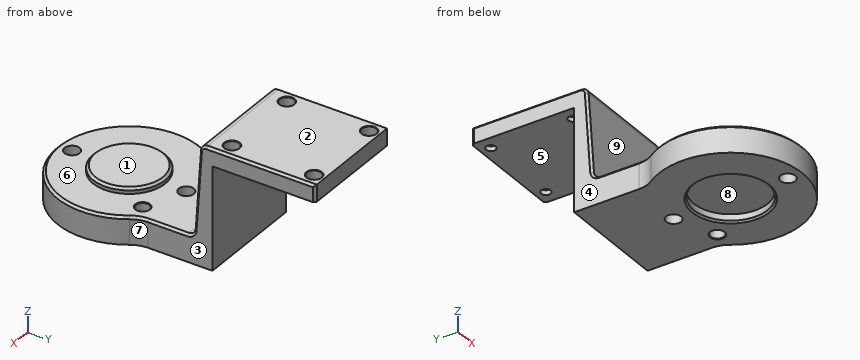
```python
from build123d import *

# Parameters (mm, degrees)
SKETCH_R          = 31.4
PAD_DEPTH         = 12
SKETCH001_R       = 16.15
PAD001_DEPTH      = 2.5
SKETCH009_R       = 15.75
PAD004_DEPTH      = 2.5
PAD001_FACE4_R    = 16.15
POCKET_DEPTH      = 3.5
SKETCH002_R       = 3.3
POCKET001_DEPTH   = 20
CHAMFER_SIZE      = 1
CHAMFER001_SIZE   = 0.75
SKETCH003_R       = 3
POCKET002_DEPTH   = 12
CHAMFER003_SIZE   = 0.25
PAD005_DEPTH      = 12
PAD006_DEPTH      = 24
PAD006_DEPTH_BACK = 24
SKETCH012_R       = 2.1
POCKET003_DEPTH   = 9.420822
SKETCH013_R       = 3.2
POCKET004_DEPTH   = 5.35
FILLET_R          = 12
FILLET001_R       = 3
CHAMFER004_SIZE   = 1
CHAMFER005_SIZE   = 1
CHAMFER006_SIZE   = 0.2


with BuildPart() as part:
    # Sketch → Pad (new body)
    with BuildSketch(Plane.XY):
        Circle(SKETCH_R)
    extrude(amount=PAD_DEPTH)

    # Sketch001 (on Sketch) → Pad001 (join)
    with BuildSketch(Plane.XY):
        Circle(SKETCH001_R)
    extrude(amount=PAD001_DEPTH)

    # Sketch009 (on Face3 of Pad001) → Pad004 (join)
    with BuildSketch(Plane.XY.offset(12)):
        Circle(SKETCH009_R)
    extrude(amount=PAD004_DEPTH)

    # Pad001 Face4 → Pocket (cut)
    with BuildSketch(Plane(origin=(0, 0, 0), x_dir=(0, -1, 0), z_dir=(0, 0, -1))):
        Circle(PAD001_FACE4_R)
    extrude(amount=-POCKET_DEPTH, mode=Mode.SUBTRACT)

    # Sketch002 → Pocket001 (cut)
    with BuildSketch(Plane.XY):
        with Locations((0, 25)):
            Circle(SKETCH002_R)
        with Locations((0, -25)):
            Circle(SKETCH002_R)
    extrude(amount=POCKET001_DEPTH, mode=Mode.SUBTRACT)

    # Chamfer
    chamfer_edges = [part.edges().sort_by_distance(p)[0] for p in [
        (-15.75, 0, 14.5),
    ]]
    chamfer(chamfer_edges, length=CHAMFER_SIZE)

    # Chamfer001
    chamfer001_edges = [part.edges().sort_by_distance(p)[0] for p in [
        (-16.15, 0, 0),
    ]]
    chamfer(chamfer001_edges, length=CHAMFER001_SIZE)

    # Sketch003 (on Face7 of Chamfer001) → Pocket002 (cut)
    with BuildSketch(Plane.XY.offset(12)):
        with Locations((17.67767, 17.67767)):
            Circle(SKETCH003_R)
    extrude(amount=-POCKET002_DEPTH, mode=Mode.SUBTRACT)

    # Chamfer003
    chamfer003_edges = [part.edges().sort_by_distance(p)[0] for p in [
        (14.67767, 17.67767, 12),
        (14.67767, 17.67767, 0),
    ]]
    chamfer(chamfer003_edges, length=CHAMFER003_SIZE)

    # Sketch011 → Pad005 (join)
    with BuildSketch(Plane.XY):
        with BuildLine():
            Line((24, 20.247469), (24, 34.174057))
            Line((24, 34.174057), (-24, 34.174057))
            Line((-24, 34.174057), (-24, 20.247469))
            ThreePointArc((24, 20.247469), (0, 31.4), (-24, 20.247469))
        make_face()
    extrude(amount=PAD005_DEPTH)

    # Sketch010 → Pad006 (join, two sides)
    with BuildSketch(Plane.YZ) as pad006_sk:
        Polygon((34.020989, 0), (52.498643, 0), (52.498643, 45), (97.498643, 45), (97.498643, 52.420822), (47.04097, 52.420822), (44.319458, 12), (34.020989, 12), align=None)
    extrude(amount=PAD006_DEPTH)
    extrude(pad006_sk.sketch, amount=-PAD006_DEPTH_BACK)

    # Sketch012 (on Face31 of Pad006) → Pocket003 (cut)
    with BuildSketch(Plane(origin=(0, 0, 45), x_dir=(1, 0, 0), z_dir=(0, 0, -1))):
        with Locations((18, -92.99873)):
            Circle(SKETCH012_R)
        with Locations((-18, -92.99873)):
            Circle(SKETCH012_R)
        with Locations((-18, -56.99873)):
            Circle(SKETCH012_R)
        with Locations((18, -56.99873)):
            Circle(SKETCH012_R)
    extrude(amount=-POCKET003_DEPTH, mode=Mode.SUBTRACT)

    # Sketch013 (on Face29 of Pocket003) → Pocket004 (cut)
    with BuildSketch(Plane.XY.offset(52.420822)):
        with Locations((18, 93.000084)):
            Circle(SKETCH013_R)
        with Locations((-18, 93.000084)):
            Circle(SKETCH013_R)
        with Locations((-18, 57.000084)):
            Circle(SKETCH013_R)
        with Locations((18, 57.000084)):
            Circle(SKETCH013_R)
    extrude(amount=-POCKET004_DEPTH, mode=Mode.SUBTRACT)

    # Fillet
    fillet_edges = [part.edges().sort_by_distance(p)[0] for p in [
        (-24, 20.247469, 6),
        (24, 20.247469, 6),
    ]]
    fillet(fillet_edges, radius=FILLET_R)

    # Fillet001
    fillet001_edges = [part.edges().sort_by_distance(p)[0] for p in [
        (0, 44.319458, 12),
        (0, 47.04097, 52.420822),
    ]]
    fillet(fillet001_edges, radius=FILLET001_R)

    # Chamfer004
    chamfer004_edges = [part.edges().sort_by_distance(p)[0] for p in [
        (24, 29.130313, 12),
        (-24, 29.130313, 12),
    ]]
    chamfer(chamfer004_edges, length=CHAMFER004_SIZE)

    # Chamfer005
    chamfer005_edges = [part.edges().sort_by_distance(p)[0] for p in [
        (24, 97.498643, 48.210411),
        (-24, 97.498643, 48.210411),
    ]]
    chamfer(chamfer005_edges, length=CHAMFER005_SIZE)

    # Chamfer006
    chamfer006_edges = [part.edges().sort_by_distance(p)[0] for p in [
        (-21.2, 57.000084, 52.420822),
        (-21.2, 93.000084, 52.420822),
        (14.8, 93.000084, 52.420822),
        (14.8, 57.000084, 52.420822),
    ]]
    chamfer(chamfer006_edges, length=CHAMFER006_SIZE)


solid = part.part
```
Input: part model. Units: mm. Frame: model coordinates. Face numbers are marked on the shaded views. A direction names the side the tool comes from. Give positions to 0.01 mm unless a question says otherwise; leave off trailing zeros. Order: outer loops, then holes, each group sorted by start corner. A loop starts at its lowest first (then second) coordinate and runs counter-clockwise, first axis right, second up. Notation, with made-up numbers: (22.5, -17) -> (26.5, -17) arc R13 cw to (26.5, 4) -> close; hole circle Ø1 at (16, 38.25). An arc over 180 degrees is marked (long way). Write each question's results on one line, items separated by ' | '. Start each with the question number.
Item 1: Cut plane A-A on y = 0. Return the cut outline in (x, z).
Item 2: Contact query for flat-ended pins moving along their axis: P1, Ø5, axis at x = 18, y = 57, coming from the -Z side; P2, Ø12, axis at x = 24.5, z = 19.5, coming from the -Y side; P3, Ø5, axis at x = 19.5, y = 56, coming from the +Z side; P4, Ø4, axis at x = -16.5, z = 17, coming from the -Y side. Output: stop coordinate, or through.
Item 3: Line query: line 1 (Y direction, x = -18, z = 50); line 2 (Z direction, x = 23, y = 12); line 3 (Y direction, x = -18, z = 45.8). Output: solid intervals per line, ascending.
Item 4: Cut plane D-D on y = 64.5. Return the cut outline in (x, z), then the cut area to 3 significant figures.
Item 5: Set-up query: the marked faces 1, 2, 3, 4 and 5. Return all of +Z, -Z, +X, -X, +Y, -Y with unobstructed straight access to the full face (end or side cutting, diameter ignored); none if empty.
Item 6: Cut plane C-C on z = 36. Return the cut outline in (x, y), then the cut area to 3 significant figures.
Item 7: Cut plane B-B on z = 6.5. Return the cut outline in (x, y), then the cut area to 3 significant figures.
Item 8: Mould query, pull axis Y, two halves, no side actions, for the marked faces 6, 7, 8 and 9. Classes: pulls with the +Y half, pulls with the -Y half, needs draft (parallel to the pull), parting line crosses it, or undercut.
Established:
1) outline: (-31.4, 0) -> (-16.9, 0) -> (-16.15, 0.75) -> (-16.15, 3.5) -> (16.15, 3.5) -> (16.15, 0.75) -> (16.9, 0) -> (31.4, 0) -> (31.4, 11) -> (30.4, 12) -> (15.75, 12) -> (15.75, 13.5) -> (14.75, 14.5) -> (-14.75, 14.5) -> (-15.75, 13.5) -> (-15.75, 12) -> (-30.4, 12) -> (-31.4, 11) -> close
2) P1: z = 45 | P2: y = 44.21 | P3: z = 52.42 | P4: y = 44.52
3) line 1: 46.9 to 53.8, 60.2 to 89.8, 96.2 to 97.5 | line 2: 0 to 12 | line 3: 46.6 to 54.9, 59.1 to 90.9, 95.1 to 97.5
4) outline: (-24, 45) -> (24, 45) -> (24, 51.42) -> (23, 52.42) -> (-23, 52.42) -> (-24, 51.42) -> close | area: 355 mm^2
5) face 1: +Z, +X, -X, -Y | face 2: +Z, +X, -X, +Y, -Y | face 3: +Z, -Z, +X, +Y | face 4: +Z, -Z, -X, +Y | face 5: -Z, +X, -X, +Y
6) outline: (-24, 46.94) -> (-23, 45.94) -> (23, 45.94) -> (24, 46.94) -> (24, 52.5) -> (-24, 52.5) -> close | area: 314 mm^2
7) outline: (-26.05, 17.54) arc R31.4 ccw (long way) to (26.05, 17.54) arc R12 cw to (24, 24.24) -> (24, 52.5) -> (-24, 52.5) -> (-24, 24.24) arc R12 cw to start; hole circle Ø6.6 at (0, -25); hole circle Ø6.6 at (0, 25); hole circle Ø6 at (17.68, 17.68) | area: 4,180 mm^2
8) face 6: undercut | face 7: pulls with the +Y half | face 8: undercut | face 9: pulls with the -Y half
